Could you check a few things on this drawing? It's one solid part, dimensions in mm from its lowest x, y, z. A direction names the side the tool comes from. Coordinates: 2 decimals unless noted, no trailing zeros. Order: outer loops, then holes, each group sorted by start corner. A loop starts at its lowest first (then second) coordinate and runs counter-clockwise, first axis right, second up. Notation, with made-up numbers: M 36,-32 L 65,-32 A26 cw 65,-4 Z; hole C 6.25,66.5 d6. An arc over 180 degrees is marked long. Answer as CSV lines item,"result". Start each with the question number.
1. On a 3-axis mill with a long thin cutter (end or side, diameter ignored), from which of +Z, -Z, +X, -X, +Y, -Y can I reach the whole of each face in a straight line? I mean the marked faces 1 and 2. Say none if no direction works.
2. If we section it at B-B (x = 31): List the corners of the cut face in (y, z) for me, plus the area to 3 significant figures.
3. I need wall thicknesses on line 1 along Y through (x, z) = (28.5, 16.75). Which ranges of the line are inside material? Lowest first, please. Write a range as from..to.
4. Will this pin go through, and if not, where does the flat tip stop? pin 1 (11 mm diameter, centred on x = 31.5, z = 17, fed in from +Y).
5. If we section it at A-A (z = 13.25): List the corners of the cut face in (x, y) for me, plus the area to 3 significant figures.
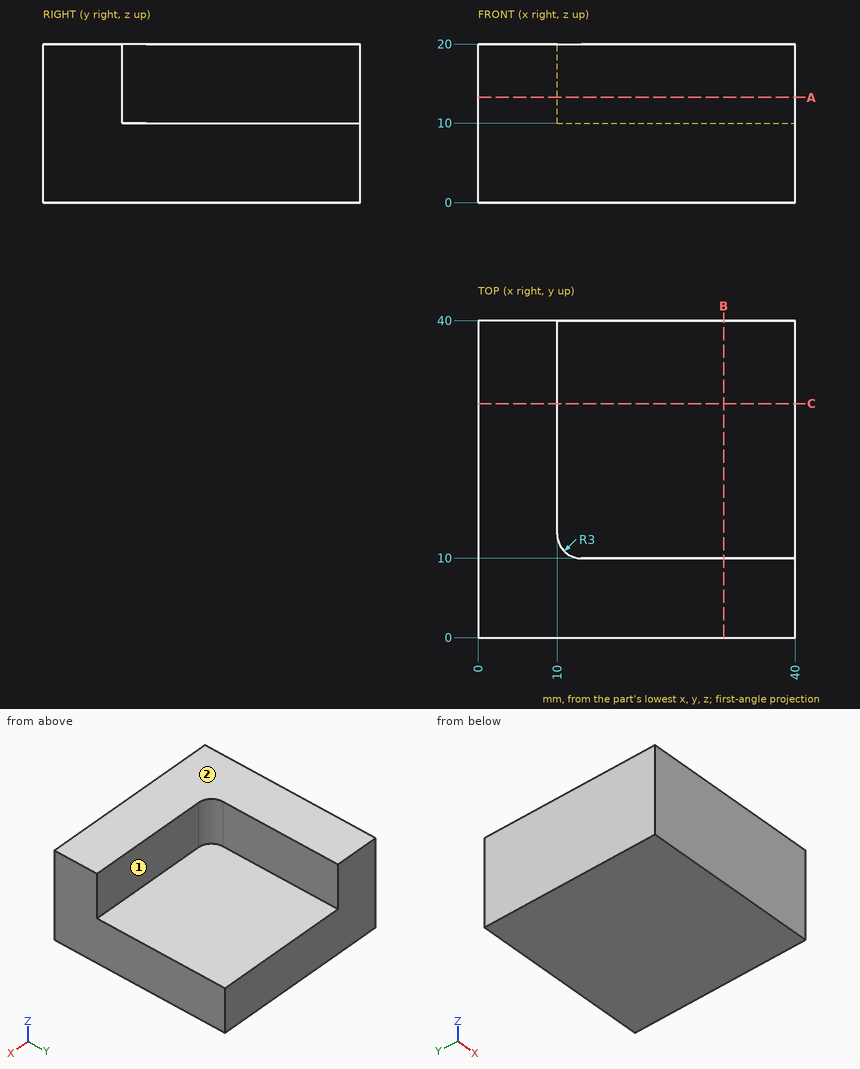
Solved:
1,face 1,"+Z, +X, +Y"
1,face 2,"+Z, +X, -X, +Y, -Y"
2,outline,"M 0,0 L 40,0 L 40,10 L 10,10 L 10,20 L 0,20 Z"
2,area,"500 mm²"
3,line 1,"0..10"
4,pin 1,"y = 10"
5,outline,"M 0,0 L 40,0 L 40,10 L 13,10 A3 cw 10,13 L 10,40 L 0,40 Z"
5,area,"702 mm²"
